from build123d import *

# Parameters (mm, degrees)
SKETCH1_W           = 70
SKETCH1_H           = 6
SKETCH2_R           = 7
BOSS_EXTRUDE1_DEPTH = 5


with BuildPart() as part:
    # Sketch1 → Revolve1 (revolve)
    with BuildSketch(Plane(origin=(0, 0, 0), x_dir=(1, 0, 0), z_dir=(0, 1, 0))):
        with Locations((0.279538905, 9)):
            Rectangle(SKETCH1_W, SKETCH1_H)
    revolve(axis=Axis((-34.720461095, 0, -6), (1, 0, 0)))

    # Sketch2 → Boss-Extrude1 (add)
    with BuildSketch(Plane.ZY.offset(34.720461095)):
        with Locations((-6, 0)):
            Circle(SKETCH2_R)
    boss_extrude1 = extrude(amount=BOSS_EXTRUDE1_DEPTH)

    # Mirror1: Boss-Extrude1 across plane
    add(boss_extrude1.mirror(Plane(origin=(0.279538905, 0, 0), x_dir=(0, 0, 1), z_dir=(1, 0, 0))))


solid = part.part
The listing builds one solid part. Answer for the finished solid, in the listing's coordinates (mm). A direction names the side the tool comes from. Give positions to 0.01 mm unless a question says otherwise; leave off trailing zeros. Write each loop counter-clockwise with the first axis right and the second up, starting at its lowest first coordinate (ties: lowest second). Pieces come first, ordered by that corner, then holes.
1) Section C-C (x = 5.5) is taken. Write down the section's boundary in (y, z), and give its area (3 significant figures).
2) Section B-B (z = -6) is taken. Write down the section's boundary in (x, y), and give its area (3 significant figures).
3) Given P1, Ø2, axis at x = -29, y = -1.5, coming from the -Z side; P2, Ø1, axis at x = -22.5, y = 2, coming from the -Z side; P3, Ø1, axis at x = 31, z = -7, coming from the +Y side, each flat-ended and moving along its own axis, determine where each tip first touches the part or whether it passes through.
4) For a pull along X with two mould halves and no side action, classify faces 1 (the face through (37.745, 2.103, 0.677)), 2 (the face through (-39.72, 0, -6)), 3 (the face through (-34.72, 2, 0)), 4 (the face through (40.28, 0, -6)) as pulls with the +X half, pulls with the -X half, needs draft (parallel to the pull), parting line crosses it, or undercut.
5) A tool of negligible diameter and unlimited length cuts with its end or side. For faces 5 (the face through (-37.185, 2.103, 0.677)), 6 (the face through (0.77, -3.65, -1.24)), from which of +Z, -Z, +X, -X, +Y, -Y can it reach the whole face along a straight path? Write none if from no direction.
6) Find the intervals of material crossed by L1, parallel to X at y = -5, z = -10; L2, parallel to Y at x = 8, z = -5.75; L3, parallel to Z at x = -9.5, y = 3.25, in increasing order.
7) Section A-A (y = 0) is taken. Write down the section's boundary in (x, z), and give its area (3 significant figures).
Response:
1. outline: circle Ø12 at (0, -6)
1. area: 113 mm2
2. outline: (-39.72, -7) - (-34.72, -7) - (-34.72, -6) - (35.28, -6) - (35.28, -7) - (40.28, -7) - (40.28, 7) - (35.28, 7) - (35.28, 6) - (-34.72, 6) - (-34.72, 7) - (-39.72, 7) - close
2. area: 980 mm2
3. P1: stops at z = -11.98
3. P2: stops at z = -11.81
3. P3: stops at y = 5.98
4. face 1: needs draft
4. face 2: pulls with the -X half
4. face 3: undercut
4. face 4: pulls with the +X half
5. face 5: +X, -X
5. face 6: none
6. L1: x = -39.72 to -34.72, 35.28 to 40.28
6. L2: y = -5.99 to 5.99
6. L3: z = -11.04 to -0.96
7. outline: (-39.72, -13) - (-34.72, -13) - (-34.72, -12) - (35.28, -12) - (35.28, -13) - (40.28, -13) - (40.28, 1) - (35.28, 1) - (35.28, 0) - (-34.72, 0) - (-34.72, 1) - (-39.72, 1) - close
7. area: 980 mm2
